For this review, take the finished solid that the model builds, in its own axes (mm). A direction names the side the tool comes from. Coordinates: 2 decimals unless noted, no trailing zeros. Loops run counter-clockwise (first coordinate to the right, second up) from the corner with the lowest first, then second, coordinate; pieces in that order, holes last. Notation, with made-up numbers: M -29,77.25 L 26,77.25 A32 cw 26,104.25 Z; hole C 56.5,-3.5 d8. An arc over 180 degrees is marked long. Use one line per item in the form item = value.
```python
from build123d import *

# Parameters (mm, degrees)
SKETCH1_R           = 12.7
BOSS_EXTRUDE1_DEPTH = 3
BOSS_EXTRUDE2_DEPTH = 12.7
CUT_EXTRUDE1_DEPTH  = 23


with BuildPart() as part:
    # Sketch1 → Boss-Extrude1 (new body)
    with BuildSketch(Plane(origin=(0, 0, 0), x_dir=(1, 0, 0), z_dir=(0, 1, 0))):
        with Locations(Location((0, 0, 0), (0, 0, 270))):
            Circle(SKETCH1_R)
    extrude(amount=BOSS_EXTRUDE1_DEPTH)

    # Sketch2 → Boss-Extrude2 (add)
    with BuildSketch(Plane(origin=(0, 3, 0), x_dir=(1, 0, 0), z_dir=(0, 1, 0))):
        Polygon((0.148889151, -5.48), (4.820263788, -2.611058213), (4.671374637, 2.868941787), (-0.148889151, 5.48), (-4.820263788, 2.611058213), (-4.671374637, -2.868941787), align=None)
    extrude(amount=BOSS_EXTRUDE2_DEPTH)

    # Sketch6 → Cut-Extrude1 (cut)
    with BuildSketch(Plane(origin=(0, 15.7, 0), x_dir=(1, 0, 0), z_dir=(0, 1, 0))):
        with BuildLine():
            Line((2.855757074, -0.919049257), (1.757975678, 2.430950743))
            ThreePointArc((1.757975678, 2.430950743), (-2.850834523, -0.934206895), (2.855757074, -0.919049257))
        make_face()
    extrude(amount=-CUT_EXTRUDE1_DEPTH, mode=Mode.SUBTRACT)


solid = part.part
```
1. Consider section D-D on x = -6.75. Write out the cut boundary in (y, z).
Computed values:
outline = M 0,-10.76 L 3,-10.76 L 3,10.76 L 0,10.76 Z
2. For pin 1 Ø1.5 at (x, y) = (5, 2.5) entering from -Z; pin 2 Ø6 at (x, y) = (-7.5, 3.5) entering from +Z; pin 3 Ø1 at (y, z) = (2, 9) entering from -X, all flat-tipped, find the tip position at first contact; note any pin that passes through.
Computed values:
pin_1 = -11.97
pin_2 = 11.86
pin_3 = -9.44
3. Consider section A-A on y = 14. Write out the cut boundary in (x, z), plus the area to 3 significant figures.
Computed values:
outline = M -4.82,-2.61 L -0.15,-5.48 L 4.67,-2.87 L 4.82,2.61 L 0.15,5.48 L -4.67,2.87 Z; hole M 1.76,-2.43 L 2.86,0.92 A3 ccw long Z
area = 51.2 mm2
4. Wall thickness on line 1 along Y through (x, z) = (-8.25, 9.5); line 2 along X through (y, z) = (5, 0); line 3 along Z through (x, y) = (0, 10.5): over which ranges is each line inside the solid? List them lowest first. Write a range as from..to.
Computed values:
line_1 = 0..3
line_2 = -4.75..-3, 2.55..4.75
line_3 = -5.4..-3, 3..5.4
5. Consider section C-C on z = -4. Write out the cut boundary in (x, y).
Computed values:
outline = M -12.05,0 L 12.05,0 L 12.05,3 L 2.58,3 L 2.58,15.7 L -2.56,15.7 L -2.56,3 L -12.05,3 Z
6. Draft analysis for pull direction Z (two halves, no side actions). For faces 4 (the face through (2.315, 7.96, -0.733)), 5 (the face through (-7.7, 1.5, -10.1)), 6 (the face through (-2.452, 9.261, -4.066)), 7 (the face through (2.1, 15.7, 2.4)), state which applies: +Z half, -Z half, draft (parallel to the pull), parting line (faces both ways), or undercut.
Computed values:
face_4 = undercut
face_5 = parting line
face_6 = -Z half
face_7 = draft
7. Consider section B-B on z = 0. Write out the cut boundary in (x, y).
Computed values:
outline = M -12.7,0 L -3,0 L -3,15.7 L -4.75,15.7 L -4.75,3 L -12.7,3 Z; M 2.55,0 L 12.7,0 L 12.7,3 L 4.75,3 L 4.75,15.7 L 2.55,15.7 Z
8. Tool access review of faces 1 (the face through (-2.29, 9.26, 4.16)), 2 (the face through (2.452, 9.261, 4.066)), 3 (the face through (-5, 3, 0)): name each direction out of +Z, -Z, +X, -X, +Y, -Y from which nothing blocks a thin tool from reaching the whole face with its end or side.
Computed values:
face_1 = +Z, -X, +Y
face_2 = +Z, +X, +Y
face_3 = +Y
